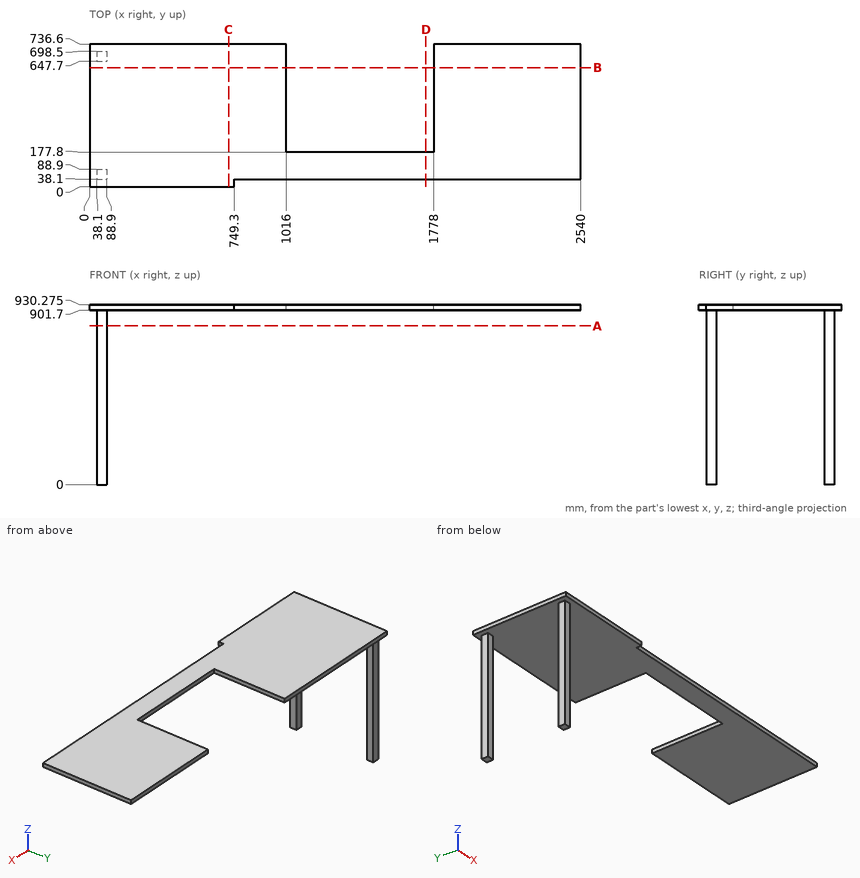
Verification items for this drawing (mm, ordinates from the low corner). Give positions to 0.01 mm unless a question says otherwise; leave off trailing zeros. Order: outer loops, then holes, each group sorted by start corner. A loop starts at its lowest first (then second) coordinate and runs counter-clockwise, first axis right, second up.
1) Cross-section at D-D (x = 1739). Record the boundary of the cut face in (y, z) (3 decimals), then the cut area to 3 significant figures.
Results are:
outline: (38.1, 901.7) - (177.8, 901.7) - (177.8, 930.275) - (38.1, 930.275) - close
area: 3,990 mm2
2) Material ranges on probe 1 along Z at (x, y) = (1916.5, 674) (3 decimals); probe 2 along X at (y, z) = (40.5, 411.5), recorded low to high.
Results are:
probe 1: z = 901.7 to 930.275
probe 2: x = 38.1 to 88.9
3) Gauge pin test, flat ends, axial feed: pin 1 (23 mm diameter, centred on x = 1575, z = 920.5, fed in from +Y); pin 2 (8.5 mm diameter, centred on y = 19, z = 909, fed in from +X). Record the tip position at first contact, or that the pin passes through.
Results are:
pin 1: stops at y = 177.8
pin 2: stops at x = 749.3
4) Cross-section at A-A (z = 819.5). Record the boundary of the cut face in (x, y), then the cut area to 3 significant figures.
Results are:
outline: (38.1, 38.1) - (88.9, 38.1) - (88.9, 88.9) - (38.1, 88.9) - close; (38.1, 647.7) - (88.9, 647.7) - (88.9, 698.5) - (38.1, 698.5) - close
area: 5,160 mm2
5) Cross-section at C-C (x = 719). Record the boundary of the cut face in (y, z) (3 decimals), then the cut area to 3 significant figures.
Results are:
outline: (0, 901.7) - (736.6, 901.7) - (736.6, 930.275) - (0, 930.275) - close
area: 21,000 mm2
6) Cross-section at B-B (y = 615). Record the boundary of the cut face in (x, z) (3 decimals).
Results are:
outline: (0, 901.7) - (1016, 901.7) - (1016, 930.275) - (0, 930.275) - close; (1778, 901.7) - (2540, 901.7) - (2540, 930.275) - (1778, 930.275) - close
